Could you check a few things on this drawing? It's one solid part, dimensions in mm from its lowest x, y, z. Coordinates: 2 decimals unless noted, no trailing zeros. Order: outer loops, then holes, each group sorted by start corner. A loop starts at its lowest first (then second) coordinate and runs counter-clockwise, first axis right, second up.
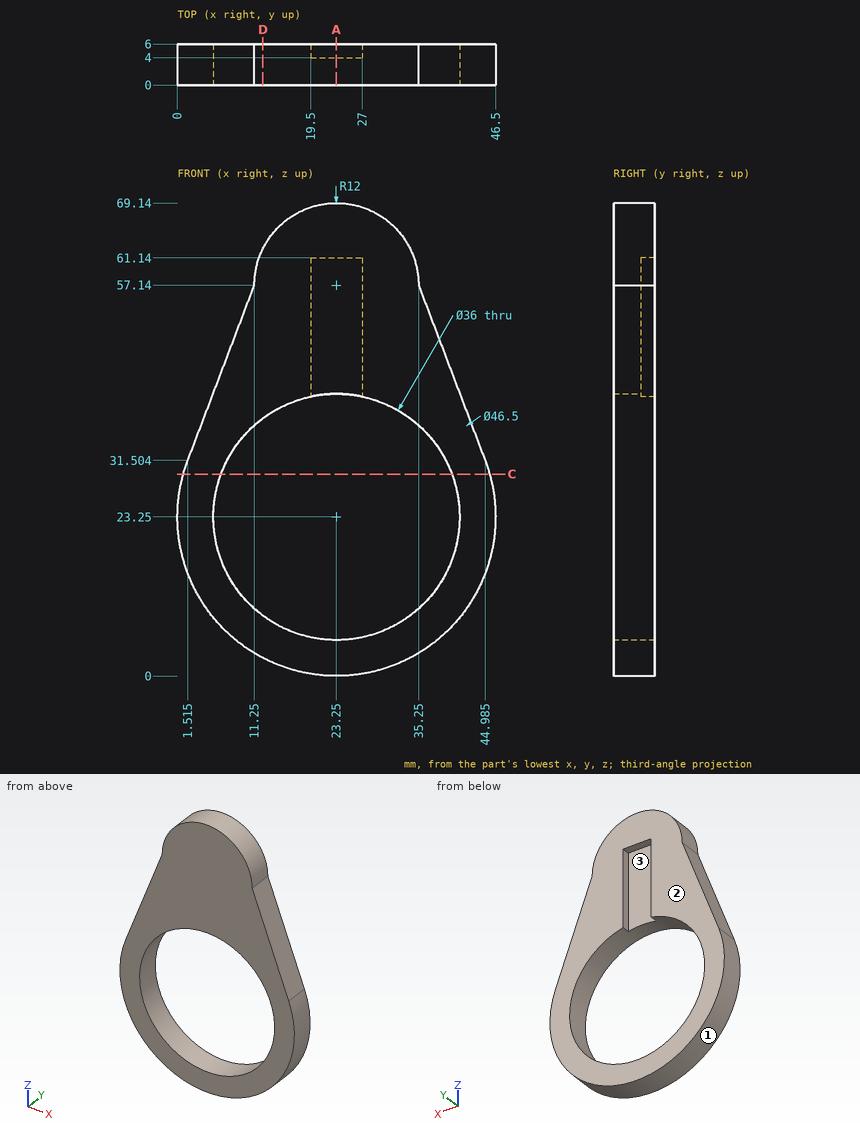
1. Please list where these lines run through material, in increasing order: probe 1 along X at (y, z) = (1.65, 23.25); probe 2 along Z at (x, y) = (16, 2.45) (1 decimal); probe 3 along X at (y, z) = (2.7, 32).
Completed:
probe 1: x = 0 to 5.25, 41.25 to 46.5
probe 2: z = 1.2 to 6.8, 39.7 to 66.7
probe 3: x = 1.7 to 7.52, 38.98 to 44.8
2. I'm going to push flat-ended pins straight in: pin 1 (2 mm diameter, centred on x = 23.5, z = 49, fed in from +Y); pin 2 (2 mm diameter, centred on y = 5.5, z = 51, fed in from -X); pin 3 (8 mm diameter, centred on x = 13.5, z = 17, fed in from -Y); pin 4 (1.6 mm diameter, centred on x = 24, y = 4.5, fed in from -Z). Where does each tip first touch, or does it pass through?
Completed:
pin 1: stops at y = 4
pin 2: stops at x = 8.54
pin 3: passes through
pin 4: stops at z = 0
3. Imagine slicing it at A-A on x = 23.25. Please give me the cut outline in (y, z), then the cut area to 3 significant figures.
Completed:
outline: (0, 0) - (6, 0) - (6, 5.25) - (0, 5.25) - close; (0, 41.25) - (4, 41.25) - (4, 61.14) - (6, 61.14) - (6, 69.14) - (0, 69.14) - close
area: 159 mm2
4. Imagine slicing it at C-C on z = 29.5. Please give me the cut outline in (x, y) (1 decimal).
Completed:
outline: (0.9, 0) - (6.4, 0) - (6.4, 6) - (0.9, 6) - close; (40.1, 0) - (45.6, 0) - (45.6, 6) - (40.1, 6) - close
5. Imagine slicing it at D-D on x = 12.5. Please give me the cut outline in (y, z) (1 decimal), then the cut area to 3 significant figures.
Completed:
outline: (0, 2.6) - (6, 2.6) - (6, 8.8) - (0, 8.8) - close; (0, 37.7) - (6, 37.7) - (6, 62.5) - (0, 62.5) - close
area: 186 mm2
6. Thinking about a two-plate mould opening in X: for the marked faces 1, 2 and 3, which applies, pulls with the +X half, pulls with the -X half, needs draft (parallel to the pull), parting line crosses it, or undercut?
Completed:
face 1: parting line crosses it
face 2: needs draft
face 3: undercut
